Input: part model. Units: mm. Frame: model coordinates. A direction names the side the tool comes from. Coordinates: 2 decimals unless noted, no trailing zeros. Loops run counter-clockwise (first coordinate to the right, second up) from the corner with the lowest first, then second, coordinate; pieces in that order, holes last. Notation, with made-up numbers: (-12, 8) - (28, 8) arc R25 ccw to (28, 32) - close; hole circle Ø10 at (15, 67.5). An arc over 180 degrees is marked (long way). Use one line per item in the form item = value.
from build123d import *

# Parameters (mm, degrees)
F0_W     = 292.1
F0_H     = 215.9
F0_W_2   = 38.1
F1_DEPTH = 2.54
F2_W     = 292.1
F2_H     = 38.1
F3_DEPTH = 2.54


with BuildPart() as f1:
    # F0 (on Top) → F1 (new body)
    with BuildSketch(Plane.XY):
        with Locations((20.573033, 78.840188)):
            Rectangle(F0_W, F0_H)
        with Locations((-144.526967, 78.840188)):
            Rectangle(F0_W_2, F0_H)
        Polygon((-125.476967, -29.109812), (-163.576967, -29.109812), (-163.576967, -67.209812), (166.623033, -67.209812), (166.623033, -29.109812), align=None)
    extrude(amount=F1_DEPTH)

    # F2 (on face) → F3 (join)
    with BuildSketch(Plane.XY.offset(2.54)):
        with Locations((20.573033, -48.159812)):
            Rectangle(F2_W, F2_H)
        Polygon((-125.476967, 186.790188), (-163.576967, 186.790188), (-163.576967, -67.209812), (-125.476967, -67.209812), (-125.476967, -29.109812), align=None)
    extrude(amount=F3_DEPTH)


solid = f1.part
Q1. Cut plane A-A, the plane x = 131. Return loops of the section in (y, z).
Check values:
outline = (-67.21, 0) - (186.79, 0) - (186.79, 2.54) - (-29.11, 2.54) - (-29.11, 5.08) - (-67.21, 5.08) - close
Q2. First-contact query: P1, Ø2, axis at y = 20.5, z = 4.5, coming from the +X side; P2, Ø10, axis at x = 6.5, y = 56.5, coming from the +Z side; P3, Ø2, axis at x = -34.5, z = 4, coming from the +Y side. Flat tips, straight axial feed; report the tip coordinate or a pass-through.
Check values:
P1 = -125.48
P2 = 2.54
P3 = -29.11
Q3. Set-up query: faces 1 (the flat face through (-1, 62, 0)), 2 (the flat face through (19, 80, 2.54)). Return all of +Z, -Z, +X, -X, +Y, -Y with unobstructed straight access to the full face (end or side cutting, diameter ignored); none if empty.
Check values:
face_1 = -Z, +X, -X, +Y, -Y
face_2 = +Z, +X, +Y
Q4. Cut plane B-B, the plane y = 29. Return loops of the section in (x, z), then the cut area to 3 significant figures.
Check values:
outline = (-163.58, 0) - (166.62, 0) - (166.62, 2.54) - (-125.48, 2.54) - (-125.48, 5.08) - (-163.58, 5.08) - close
area = 935 mm²
Q5. Ray query, line 1 along Z through (x, y) = (128.5, 161.5); line 2 along Y through (x, z) = (122.5, 4.05); line 3 along X through (y, z) = (14, 3.05). Return the intervals inside material, ascending. Write a range as [from, to].
Check values:
line_1 = [0, 2.54]
line_2 = [-67.21, -29.11]
line_3 = [-163.58, -125.48]
